```python
from build123d import *

# Parameters (mm, degrees)
F0_W     = 508
F0_H     = 609.6
F1_DEPTH = 19.05
F3_DEPTH = 19.05
F5_DEPTH = 19.05
F6_W     = 609.6
F6_H     = 387.35
F7_DEPTH = 19.05


with BuildPart() as f1:
    # F0 (on Top) → F1 (new body)
    with BuildSketch(Plane.XY):
        Rectangle(F0_W, F0_H)
    extrude(amount=F1_DEPTH)

    # F2 (on face) → F3 (join)
    with BuildSketch(Plane.XZ.offset(304.8)):
        Polygon((-230.1875, 19.05), (254, 19.05), (254, 406.4), align=None)
        Polygon((-254, 0), (254, 0), (254, 19.05), (-230.1875, 19.05), align=None)
    extrude(amount=F3_DEPTH)

    # F4 (on face) → F5 (join)
    with BuildSketch(Plane(origin=(0, 304.8, 0), x_dir=(-1, 0, 0), z_dir=(0, 1, 0))):
        Polygon((-254, 406.4), (-254, 19.05), (230.1875, 19.05), align=None)
        Polygon((-254, 19.05), (-254, 0), (254, 0), (230.1875, 19.05), align=None)
    extrude(amount=F5_DEPTH)

    # F6 (on face) → F7 (join)
    with BuildSketch(Plane.YZ.offset(254)):
        with Locations((0, 212.725)):
            Rectangle(F6_W, F6_H)
        Polygon((-323.85, 0), (323.85, 0), (323.85, 406.4), (304.8, 406.4), (304.8, 19.05), (-304.8, 19.05), (-304.8, 406.4), (-323.85, 406.4), align=None)
    extrude(amount=F7_DEPTH)


solid = f1.part
```
Can you work these out from the model? Positions are in its coordinate system, mm. A direction names the side the tool comes from. Give positions to 0.01 mm unless a question says otherwise; leave off trailing zeros. Loops run counter-clockwise (first coordinate to the right, second up) from the corner with the lowest first, then second, coordinate; pieces in that order, holes last. Notation, with made-up numbers: M 11,-23 L 22,-23 A17 cw 22,10 Z; hole C -14,14 d1. An arc over 180 degrees is marked long. Use CSV: the item, a comma, the result in double quotes. Start each with the question number.
1. Imagine slicing it at C-C, the plane y = 188. Write out the boundary of the cut face in (x, z).
2. On a 3-axis mill with a long thin cutter (end or side, diameter ignored), from which of +Z, -Z, +X, -X, +Y, -Y can I reach the whole of each face in a straight line? I mean faces 4 (the face through (-248, 304.8, 14)), 5 (the face through (123, 304.8, 129)), 6 (the face through (-254, -4, 9)). Say none if no direction works.
3. For P1, Ø6, axis at x = 109.5, y = -9, coming from the +Z side; P2, Ø8, axis at y = -135.5, z = 183.5, coming from the -X side; P3, Ø8, axis at x = -181, y = -239, coming from the -Z side; P4, Ø5.5, axis at x = -248, z = 9.5, coming from the +Y side, each with a flat end and sliding along its axis, tell me the tip position at first contact or that it passes through.
4. If I drill on L1, parallel to Y at x = -32.5, z = 177; L2, parallel to X at y = 76, z = 382; L3, parallel to Z at x = 82, y = 70.5, over which ranges is the centre line in solid material (lowest first)?
5. Imagine slicing it at B-B, the plane z = 252. Write out the boundary of the cut face in (x, y), plus the area to 3 significant figures.
6. If we mould it in two halves opening along Z, with no side actions, what happens to faces 1 (the face through (6, -5, 0)), 2 (the face through (3.556, -314.192, 206.045)), 3 (the face through (-248, -304.8, 14))? For each: released by +Z, released by -Z, zero draft, split by the parting line, or undercut.
7. Imagine slicing it at A-A, the plane x = 133.5. Write out the boundary of the cut face in (y, z), plus the area to 3 significant figures.
Response values:
1,outline,"M -254,0 L 273.05,0 L 273.05,406.4 L 254,406.4 L 254,19.05 L -254,19.05 Z"
2,face 4,"+Z, -X, +Y"
2,face 5,"+Z, -X"
2,face 6,"+Z, -Z, -X, +Y, -Y"
3,P1,"z = 19.05"
3,P2,"x = 254"
3,P3,"z = 0"
3,P4,"y = 304.8"
4,L1,"-323.85 to -304.8, 304.8 to 323.85"
4,L2,"254 to 273.05"
4,L3,"0 to 19.05"
5,outline,"M 61,-323.85 L 273.05,-323.85 L 273.05,323.85 L 61,323.85 L 61,304.8 L 254,304.8 L 254,-304.8 L 61,-304.8 Z"
5,area,"19,700 mm^2"
6,face 1,"released by -Z"
6,face 2,"released by +Z"
6,face 3,"zero draft"
7,outline,"M -323.85,0 L 323.85,0 L 323.85,310 L 304.8,310 L 304.8,19.05 L -304.8,19.05 L -304.8,310 L -323.85,310 Z"
7,area,"23,400 mm^2"
